Part model, mm, in its own coordinate system. A direction names the side the tool comes from. Give positions to 0.01 mm unless a question says otherwise; leave off trailing zeros. Order: outer loops, then holes, each group sorted by start corner. A loop starts at its lowest first (then second) coordinate and runs counter-clockwise, first axis right, second up. Notation, with made-up numbers: (54.5, 59.25) - (73.5, 59.25) arc R18 ccw to (73.5, 92.25) - close; hole circle Ø8 at (54, -39). An arc over 180 degrees is marked (long way). One line per item, written item: value.
```python
from build123d import *

# Parameters (mm, degrees)
SKETCH1_R           = 7.5
BOSS_EXTRUDE1_DEPTH = 30
SKETCH1_4_R         = 35
SKETCH1_4_R_2       = 10
BOSS_EXTRUDE2_DEPTH = 20
BOSS_EXTRUDE3_START = -50
SKETCH1_5_R         = 35
SKETCH1_5_R_2       = 10
BOSS_EXTRUDE3_DEPTH = 20
SKETCH1_6_R         = 10
BOSS_EXTRUDE4_DEPTH = 70
BOSS_EXTRUDE5_START = -100
SKETCH1_7_R         = 10
BOSS_EXTRUDE5_DEPTH = 70


with BuildPart() as part:
    # Sketch1 → Boss-Extrude1 (new body)
    with BuildSketch(Plane.XY):
        with Locations((0, 25)):
            Circle(SKETCH1_R)
    extrude(amount=-BOSS_EXTRUDE1_DEPTH)

    # Sketch1<4> → Boss-Extrude2 (add)
    with BuildSketch(Plane.XY):
        Circle(SKETCH1_4_R)
        Circle(SKETCH1_4_R_2, mode=Mode.SUBTRACT)
    extrude(amount=BOSS_EXTRUDE2_DEPTH)

    # Sketch1<5> → Boss-Extrude3 (add)
    with BuildSketch(Plane.XY.offset(BOSS_EXTRUDE3_START)):
        Circle(SKETCH1_5_R)
        Circle(SKETCH1_5_R_2, mode=Mode.SUBTRACT)
    extrude(amount=BOSS_EXTRUDE3_DEPTH)

    # Sketch1<6> → Boss-Extrude4 (add)
    with BuildSketch(Plane.XY):
        Circle(SKETCH1_6_R)
    extrude(amount=BOSS_EXTRUDE4_DEPTH)

    # Sketch1<7> → Boss-Extrude5 (add)
    with BuildSketch(Plane.XY.offset(BOSS_EXTRUDE5_START)):
        Circle(SKETCH1_7_R)
    extrude(amount=BOSS_EXTRUDE5_DEPTH)


solid = part.part
```
1) Cut at A-A, the plane y = 0. Give the cut face in (x, z), then the cut area to 3 significant figures.
Outcome:
outline: (-35, -50) - (-10, -50) - (-10, -100) - (10, -100) - (10, -50) - (35, -50) - (35, -30) - (-35, -30) - close; (-35, 0) - (35, 0) - (35, 20) - (10, 20) - (10, 70) - (-10, 70) - (-10, 20) - (-35, 20) - close
area: 4,800 mm^2
2) Drill centre lines: line 1 along Z through (x, y) = (4.5, -3); line 2 along Z through (x, y) = (-18.5, -27); line 3 along Y through (x, z) = (0, -65). Where is each one in solid material? Low to high. Write a range as from..to.
Outcome:
line 1: z = -100..-30, 0..70
line 2: z = -50..-30, 0..20
line 3: y = -10..10
3) Cut at B-B, the plane x = 20.5. Give the cut face in (y, z).
Outcome:
outline: (-28.37, -50) - (28.37, -50) - (28.37, -30) - (-28.37, -30) - close; (-28.37, 0) - (28.37, 0) - (28.37, 20) - (-28.37, 20) - close
4) Cut at D-D, the plane y = 25. Give the cut face in (x, z), then the cut area to 3 significant figures.
Outcome:
outline: (-24.49, -50) - (24.49, -50) - (24.49, -30) - (7.5, -30) - (7.5, 0) - (24.49, 0) - (24.49, 20) - (-24.49, 20) - (-24.49, 0) - (-7.5, 0) - (-7.5, -30) - (-24.49, -30) - close
area: 2,410 mm^2
5) Which spindle directions (+Z, -Z, +X, -X, +Y, -Y) get a long thin tool onto all of the face, cutting with end or side? Do faces 1 (the cylindrical face through (-28, -21, 10)), 2 (the flat face through (7.3, -7.3, -50)), 3 (the cylindrical face through (-2.17, -9.76, 44.65)), 4 (the cylindrical face through (-0.976, 32.436, -14.79)). Say none if no direction does.
Outcome:
face 1: +Z, -Z
face 2: -Z
face 3: +Z
face 4: none
6) Mould opens along Z. For faces 5 (the flat face through (0, 0, -30)), 6 (the flat face through (0, 0, 70)), 7 (the cylindrical face through (-2.17, -9.76, -75.35)) say: released by +Z, released by -Z, zero draft, split by the parting line, or undercut.
Outcome:
face 5: undercut
face 6: released by +Z
face 7: zero draft
7) Pin check, flat tips, straight feed: pin 1 (10 mm diameter, centred on x = -5, y = 27, fed in from -Z); pin 2 (10 mm diameter, centred on x = 9.5, z = -35.5, fed in from -Y); pin 3 (12 mm diameter, centred on x = 7.5, z = 38, fed in from -Y); pin 4 (21 mm diameter, centred on x = -12, y = 13.5, fed in from -Z). Stop position of each tip, or through.
Outcome:
pin 1: stops at z = -50
pin 2: stops at y = -34.71
pin 3: stops at y = -9.89
pin 4: stops at z = -100
8) Cut at C-C, the plane x = 0. Give the cut face in (y, z).
Outcome:
outline: (-35, -50) - (-10, -50) - (-10, -100) - (10, -100) - (10, -50) - (35, -50) - (35, -30) - (32.5, -30) - (32.5, 0) - (35, 0) - (35, 20) - (10, 20) - (10, 70) - (-10, 70) - (-10, 20) - (-35, 20) - (-35, 0) - (17.5, 0) - (17.5, -30) - (-35, -30) - close
